The figure shows three views and two pictorial views of one solid part (mm, origin at its lowest corner). Answer the questions. A direction names the side the tool comes from. Coordinates: 2 decimals unless noted, no trailing zeros. Write each loop counter-clockwise with the first axis right and the second up, starting at its lowest first coordinate (ties: lowest second). Pieces come first, ordered by that corner, then holes. Notation, with made-up numbers: M 65.5,-0.5 L 84.5,-0.5 A21 ccw 84.5,9.5 Z; hole C 85,46 d9. An arc over 180 degrees is marked long. Use CSV: the item, a comma, the result in double quotes.
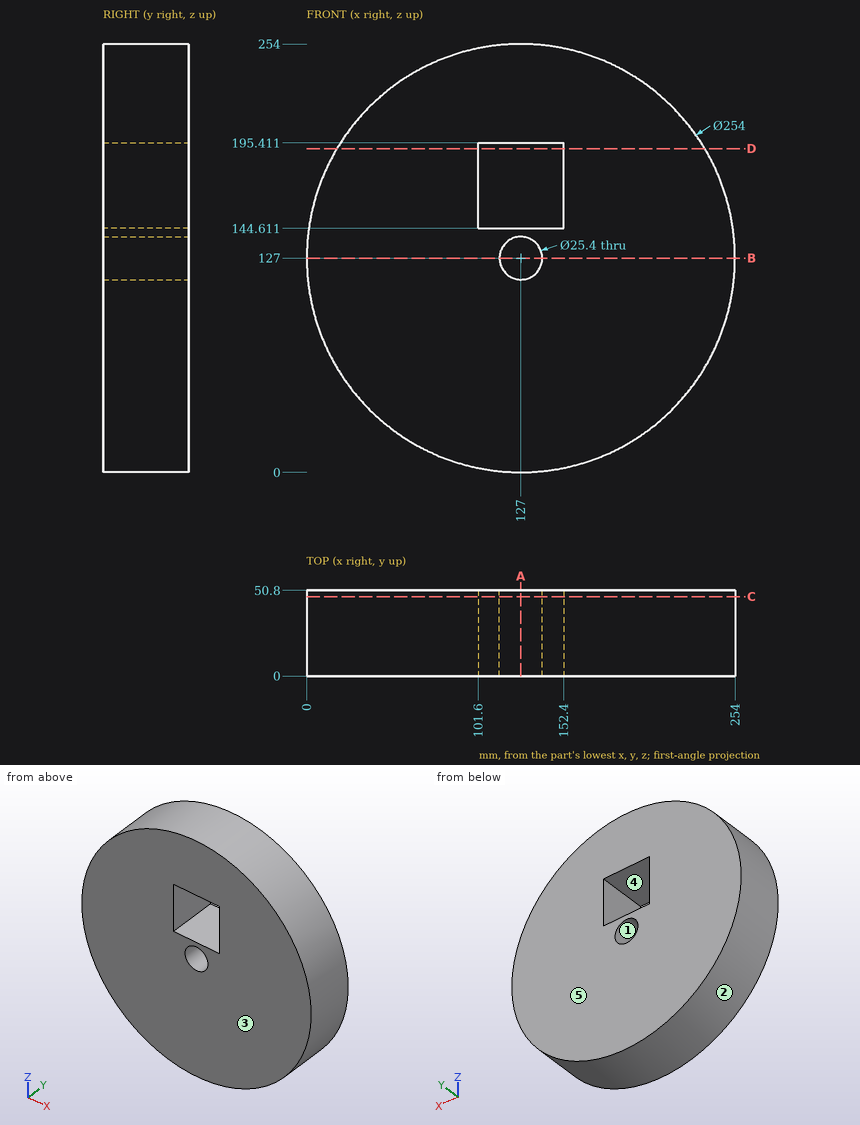
Item 1: The part is cut by section A-A (x = 127). Write down the section's boundary in (y, z), then the cut area to 3 significant figures.
Answer:
outline,"M 0,0 L 50.8,0 L 50.8,114.3 L 0,114.3 Z; M 0,139.7 L 50.8,139.7 L 50.8,144.61 L 0,144.61 Z; M 0,195.41 L 50.8,195.41 L 50.8,254 L 0,254 Z"
area,"9,030 mm2"
Item 2: For a pull along X with two mould halves and no side action, classify the marked faces 1, 2 and 3 as released by +X, released by -X, zero draft, split by the parting line, or undercut.
Answer:
face 1,"undercut"
face 2,"split by the parting line"
face 3,"zero draft"
Item 3: Consider probe 1 along Z at (x, y) = (127, 24); probe 2 along Z at (x, y) = (135.5, 37.5) (1 decimal); probe 3 along Z at (x, y) = (140, 22). Determine where each line is inside the solid, lowest interval first.
Answer:
probe 1,"z = 0 to 114.3, 139.7 to 144.61, 195.41 to 254"
probe 2,"z = 0.3 to 117.6, 136.4 to 144.6, 195.4 to 253.7"
probe 3,"z = 0.67 to 144.61, 195.41 to 253.33"
Item 4: The part is cut by section D-D (z = 192). Write down the section's boundary in (x, y) (1 decimal), then the cut area to 3 significant figures.
Answer:
outline,"M 17.9,0 L 101.6,0 L 101.6,50.8 L 17.9,50.8 Z; M 152.4,0 L 236.1,0 L 236.1,50.8 L 152.4,50.8 Z"
area,"8,500 mm2"
Item 5: The part is cut by section B-B (z = 127). Write down the section's boundary in (x, y), then the cut area to 3 significant figures.
Answer:
outline,"M 0,0 L 114.3,0 L 114.3,50.8 L 0,50.8 Z; M 139.7,0 L 254,0 L 254,50.8 L 139.7,50.8 Z"
area,"11,600 mm2"
Item 6: Given pin 1 (4 mm diameter, centred on x = 203, y = 31, fed in from -Z); pin 2 (2 mm diameter, centred on y = 20.5, z = 68, fed in from -X); pin 3 (12 mm diameter, centred on y = 36, z = 123, fed in from -X); pin 4 (8 mm diameter, centred on y = 34, z = 165.5, fed in from -X), each flat-ended and moving along its own axis, determine where each tip first touches the part or whether it passes through.
Answer:
pin 1,"stops at z = 23.79"
pin 2,"stops at x = 14.02"
pin 3,"stops at x = 0"
pin 4,"stops at x = 4.78"
Item 7: A tool of negligible diameter and unlimited length cuts with its end or side. For the marked faces 4 and 5, from which of +Z, -Z, +X, -X, +Y, -Y can it reach the whole face along a straight path? Write none if from no direction.
Answer:
face 4,"+Y, -Y"
face 5,"+Z, -Z, +X, -X, +Y"
Item 8: The part is cut by section C-C (y = 47). Write down the section's boundary in (x, z).
Answer:
outline,"C 127,127 d254; hole M 101.6,144.61 L 152.4,144.61 L 152.4,195.41 L 101.6,195.41 Z; hole C 127,127 d25.4"
